Part print with two shaded views. Sizes in mm from the minimum x, y, z corner. A direction names the side the tool comes from. Coordinates: 2 decimals unless noted, no trailing zeros. Order: outer loops, then holes, each group sorted by start corner. A loop starts at its lowest first (then second) coordinate and runs counter-clockwise, first axis right, second up. Notation, with made-up numbers: (85, 12) - (139, 12) arc R23 cw to (139, 39) - close; hole circle Ø7 at (60.25, 54). An arc over 180 degrees is marked (long way). Write each question's results on one line, items separated by ' | '. Start each with the question number.
Q1. Band-saw the part on D-D, the plane y = 17. Write the cut outline in (x, z) (3 decimals), then the cut area to 3 significant figures.
Q2. Band-saw the part on C-C, the plane z = 123. Write the cut outline in (x, y), then the cut area to 3 significant figures.
Q3. Which spindle directions (+Z, -Z, +X, -X, +Y, -Y) get a long thin tool onto all of the face, cutting with end or side? Do the marked faces 1 and 2. Say none if no direction does.
Q4. Band-saw the part on A-A, the plane x = 30.4. Write the cut outline in (y, z) (3 decimals), then the cut area to 3 significant figures.
Q5. Pin check, flat tips, straight feed: P1, Ø10, axis at y = 25.5, z = 17, coming from the +X side; P2, Ø1.5, axis at y = 34, z = 17, coming from the +X side; P3, Ø12, axis at x = 38, z = 36.5, coming from the -Y side; P4, Ø18, axis at x = 38.5, y = 35.5, coming from the -Z side. Stop position of each tip, or through.
Q6. Wall check: probe 1 along Z at (x, y) = (28, 49) (3 decimals); probe 2 along Y at (x, z) = (31, 154); probe 3 along Z at (x, y) = (17.5, 34) (3 decimals). Give the ranges that are in metal, low to high.
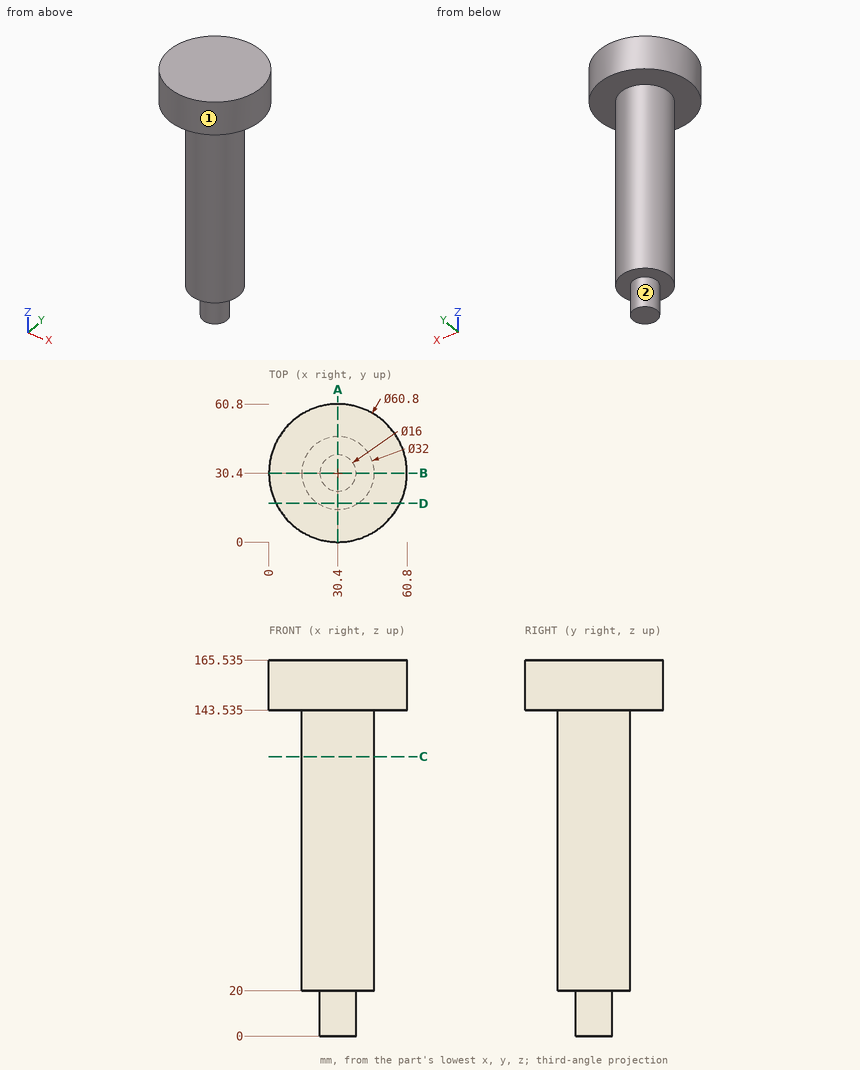
Results below:
1) outline: (3.113, 143.535) - (21.657, 143.535) - (21.657, 20) - (39.143, 20) - (39.143, 143.535) - (57.687, 143.535) - (57.687, 165.535) - (3.113, 165.535) - close | area: 3,360 mm²
2) outline: circle Ø32 at (30.4, 30.4) | area: 804 mm²
3) face 1: +Z, -Z | face 2: -Z
4) outline: (0, 143.535) - (14.4, 143.535) - (14.4, 20) - (22.4, 20) - (22.4, 0) - (38.4, 0) - (38.4, 20) - (46.4, 20) - (46.4, 143.535) - (60.8, 143.535) - (60.8, 165.535) - (0, 165.535) - close | area: 5,610 mm²
5) P1: stops at x = 46.37 | P2: stops at x = 37.88 | P3: stops at y = 14.48 | P4: stops at z = 0
6) probe 1: z = 143.535 to 165.535 | probe 2: y = 0.01 to 60.79 | probe 3: z = 20 to 165.535
